Can you work these out from the drawing? Everything is in mm from the part's minimum corner. Coordinates: 2 decimals unless noted, no trailing zeros. Order: outer loops, then holes, each group sorted by start corner. A loop starts at its lowest first (then second) coordinate and runs counter-clockwise, first axis right, second up. Notation, with made-up numbers: (-15.75, 82) - (11.25, 82) arc R32 cw to (11.25, 109) - close; hole circle Ø6 at (-11, 56.25). An arc over 180 degrees is marked (long way). One line per item, written item: value.
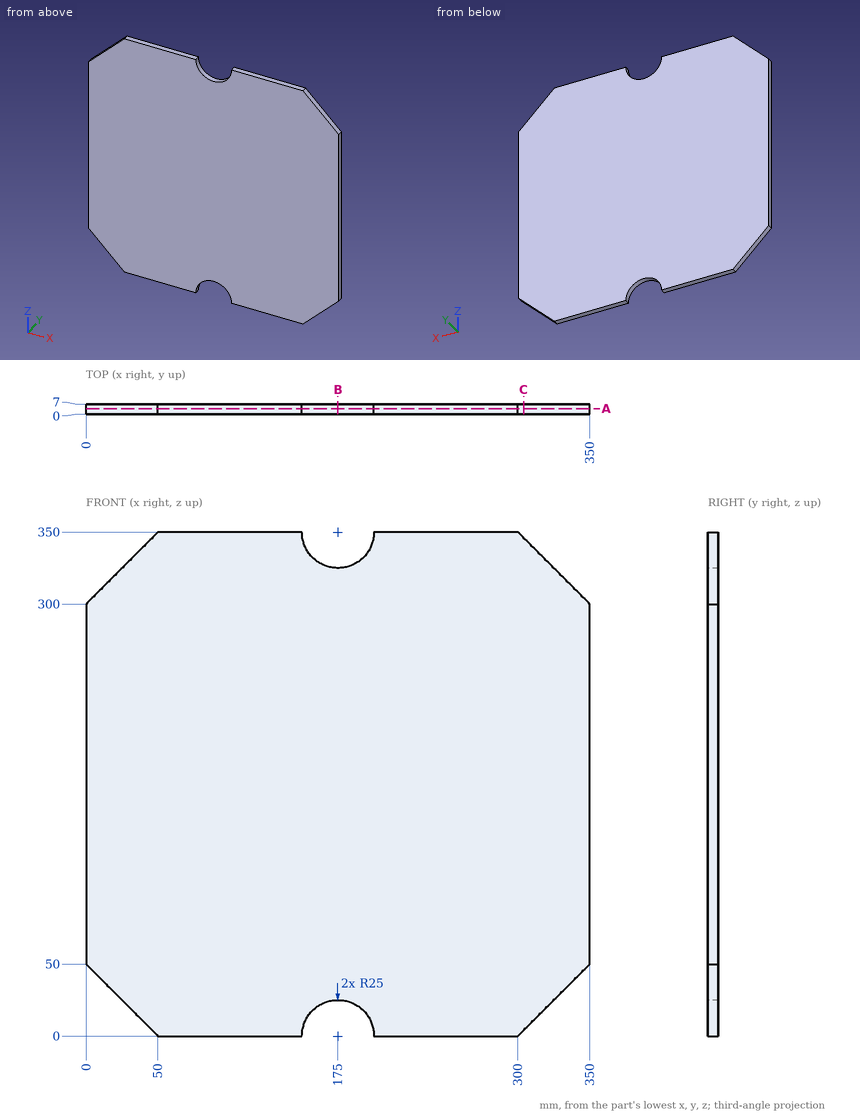
Item 1: If I drill on probe 1 along X at (y, z) = (2.5, 332); probe 2 along Z at (x, y) = (193, 3.75); probe 3 along Z at (x, y) = (48.5, 6.75), over which ranges is the centre line in solid material (lowest first)?
Conclusion:
probe 1: 32 to 157.65, 192.35 to 318
probe 2: 17.35 to 332.65
probe 3: 1.5 to 348.5
Item 2: I'm going to push a flat-ended pin straight in: pin 1 Ø4 at (y, z) = (2.5, 42) entering from +X. Where does the tip first touch, or does it pass through?
Conclusion:
pin 1: x = 344
Item 3: I want a section at B-B on x = 175. Please give me the cut outline in (y, z), then the cut area to 3 significant figures.
Conclusion:
outline: (0, 25) - (7, 25) - (7, 325) - (0, 325) - close
area: 2,100 mm²
Item 4: I want a section at C-C on x = 304. Please give me the cut outline in (y, z).
Conclusion:
outline: (0, 4) - (7, 4) - (7, 346) - (0, 346) - close
Item 5: I want a section at A-A on y = 3.75. Please give me the cut outline in (x, z), then the cut area to 3 significant figures.
Conclusion:
outline: (0, 50) - (50, 0) - (150, 0) arc R25 cw to (200, 0) - (300, 0) - (350, 50) - (350, 300) - (300, 350) - (200, 350) arc R25 cw to (150, 350) - (50, 350) - (0, 300) - close
area: 116,000 mm²
